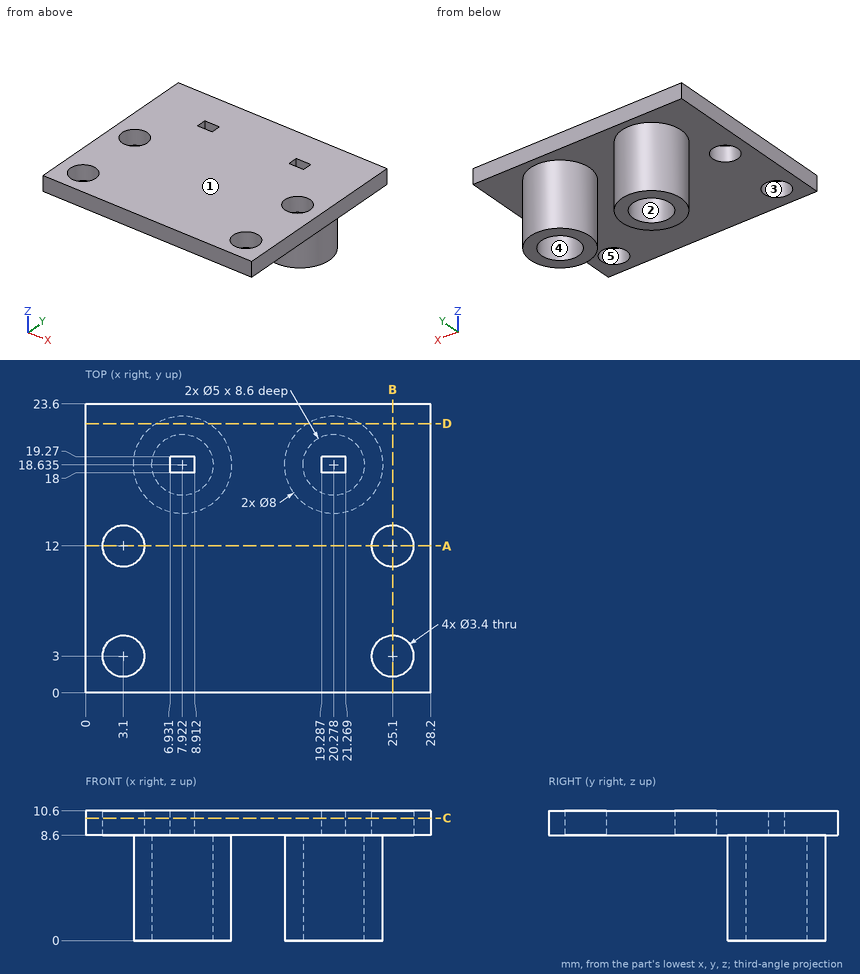
Verification items for this drawing (mm, ordinates from the low corner). A direction names the side the tool comes from. Coordinates: 2 decimals unless noted, no trailing zeros. Order: outer loops, then holes, each group sorted by start corner. A loop starts at its lowest first (then second) coordinate and runs counter-clockwise, first axis right, second up.
Q1. Sectioned sample at B-B on x = 25.1. Record the cut outline in (y, z), and give its area (3 significant figures).
Reply:
outline: (0, 8.6) - (1.3, 8.6) - (1.3, 10.6) - (0, 10.6) - close; (4.7, 8.6) - (10.3, 8.6) - (10.3, 10.6) - (4.7, 10.6) - close; (13.7, 8.6) - (23.6, 8.6) - (23.6, 10.6) - (13.7, 10.6) - close
area: 33.6 mm2
Q2. Thickness scan on probe 1 along Y at (x, z) = (3.1, 9.15); probe 2 along X at (y, z) = (18.75, 8) (1 decimal); probe 3 along X at (y, z) = (19.75, 6.25) (1 decimal). Record the ranges inside material, lowest first.
Reply:
probe 1: y = 0 to 1.3, 4.7 to 10.3, 13.7 to 23.6
probe 2: x = 3.9 to 5.4, 10.4 to 11.9, 16.3 to 17.8, 22.8 to 24.3
probe 3: x = 4.1 to 5.7, 10.2 to 11.8, 16.4 to 18, 22.5 to 24.1
Q3. Tool access check on the marked faces 4 and 5. Record the directions out of +Z, -Z, +X, -X, +Y, -Y that give a thin tool (end or side, any length) a straight path to the whole face; none if there is none.
Reply:
face 4: -Z
face 5: +Z, -Z
Q4. Sectioned sample at D-D on y = 22. Record the cut outline in (x, z) (1 decimal), and give its area (3 significant figures).
Reply:
outline: (0, 8.6) - (5.8, 8.6) - (5.8, 0) - (10.1, 0) - (10.1, 8.6) - (18.1, 8.6) - (18.1, 0) - (22.4, 0) - (22.4, 8.6) - (28.2, 8.6) - (28.2, 10.6) - (0, 10.6) - close
area: 131 mm2
Q5. Sectioned sample at C-C on z = 10. Record the cut outline in (x, y), and give its area (3 significant figures).
Reply:
outline: (0, 0) - (28.2, 0) - (28.2, 23.6) - (0, 23.6) - close; hole circle Ø3.4 at (3.1, 3); hole circle Ø3.4 at (3.1, 12); hole (6.93, 18) - (8.91, 18) - (8.91, 19.27) - (6.93, 19.27) - close; hole (19.29, 18) - (21.27, 18) - (21.27, 19.27) - (19.29, 19.27) - close; hole circle Ø3.4 at (25.1, 3); hole circle Ø3.4 at (25.1, 12)
area: 624 mm2
Q6. Draft check along X on the marked faces 1, 2 and 3. Enter one of: released by +X, released by -X, zero draft, split by the parting line, or undercut.
Reply:
face 1: zero draft
face 2: undercut
face 3: undercut
Q7. Depth check by flat-ended pin: pin 1 Ø2 at (x, y) = (3.1, 3) entering from -Z; pin 2 Ø8 at (x, y) = (23.5, 6.5) entering from -Z; pin 3 Ø5 at (x, z) = (24.5, 2) entering from +Y (1 decimal); pin 4 Ø3 at (x, z) = (9, 3) entering from +Y (1 decimal). Enter the tip coordinate at first touch or a pass-through.
Reply:
pin 1: passes through
pin 2: stops at z = 8.6
pin 3: stops at y = 22.2
pin 4: stops at y = 22.6
Q8. Sectioned sample at A-A on y = 12. Record the cut outline in (x, z).
Reply:
outline: (0, 8.6) - (1.4, 8.6) - (1.4, 10.6) - (0, 10.6) - close; (4.8, 8.6) - (23.4, 8.6) - (23.4, 10.6) - (4.8, 10.6) - close; (26.8, 8.6) - (28.2, 8.6) - (28.2, 10.6) - (26.8, 10.6) - close
